```python
from build123d import *

# Parameters (mm, degrees)
SKETCH_1_W                  = 82
SKETCH_1_H                  = 160
EXTRUDE_1_DEPTH             = 50
SKETCH_2_W                  = 79.5
SKETCH_2_H                  = 47.5
CUT_EXTRUDE_1_DEPTH         = 187.611896727
CUT_EXTRUDE_6_DEPTH         = 186.95765647
CUT_EXTRUDE_9_DEPTH         = 187.611896727
CUT_EXTRUDE_10_DEPTH        = 187.611896727
CUT_EXTRUDE_11_DEPTH        = 187.611896727
CUT_EXTRUDE_12_DEPTH        = 187.611896727
CUT_EXTRUDE_13_DEPTH        = 187.611896727
CUT_EXTRUDE_14_DEPTH        = 187.611896727
CUT_EXTRUDE_15_DEPTH        = 187.611896727
CUT_EXTRUDE_16_DEPTH        = 187.611896727
CUT_EXTRUDE_17_DEPTH        = 187.611896727
CUT_EXTRUDE_18_DEPTH        = 187.611896727
CUT_EXTRUDE_19_DEPTH        = 187.611896727
CUT_EXTRUDE_20_DEPTH        = 187.611896727
HOLE_WIZARD_3_4_3_4_1_D     = 3.4
HOLE_WIZARD_3_4_3_4_1_DEPTH = 50
HOLE_WIZARD_3_2_3_2_2_D     = 3.2
HOLE_WIZARD_3_2_3_2_2_DEPTH = 82
HOLE_WIZARD_5_0_5_1_D       = 5
HOLE_WIZARD_5_0_5_1_DEPTH   = 50
FILLET_1_R                  = 0.5
FILLET_2_R                  = 2
FILLET_3_R                  = 5
SKETCH_30_R                 = 1.6
CUT_EXTRUDE_21_DEPTH        = 10
SKETCH_31_R                 = 1.6
CUT_EXTRUDE_22_DEPTH        = 186.52695222


with BuildPart() as part:
    # 草图1 → 凸台-拉伸1 (new body)
    with BuildSketch(Plane(origin=(0, 0, -50), x_dir=(-1, 0, 0), z_dir=(0, 0, -1))):
        with Locations((-41, 80)):
            Rectangle(SKETCH_1_W, SKETCH_1_H)
    extrude(amount=-EXTRUDE_1_DEPTH)

    # 草图2 → 切除-拉伸1 (cut, through all)
    with BuildSketch(Plane(origin=(0, 160, 0), x_dir=(-1, 0, 0), z_dir=(0, 1, 0))):
        with Locations((-39.75, -26.25)):
            Rectangle(SKETCH_2_W, SKETCH_2_H)
    extrude(amount=-CUT_EXTRUDE_1_DEPTH, mode=Mode.SUBTRACT)

    # 草图7 → 切除-拉伸6 (cut, through all)
    with BuildSketch(Plane(origin=(0, 0, -2.5), x_dir=(-1, 0, 0), z_dir=(0, 0, -1))):
        with BuildLine():
            Line((-68, 20), (-38, 20))
            ThreePointArc((-38, 20), (-36.4, 21.6), (-38, 23.2))
            Line((-38, 23.2), (-68, 23.2))
            ThreePointArc((-68, 23.2), (-69.6, 21.6), (-68, 20))
        make_face()
    extrude(amount=-CUT_EXTRUDE_6_DEPTH, mode=Mode.SUBTRACT)

    # 草图10 → 切除-拉伸9 (cut, through all)
    with BuildSketch(Plane(origin=(82, 0, 0), x_dir=(0, 0, -1), z_dir=(1, 0, 0))):
        with BuildLine():
            Line((20.690598923, 80), (16.690598923, 86.92820323))
            ThreePointArc((16.690598923, 86.92820323), (13.629378785, 80), (16.690598923, 73.07179677))
            Line((16.690598923, 73.07179677), (20.690598923, 80))
        make_face()
    extrude(amount=-CUT_EXTRUDE_9_DEPTH, mode=Mode.SUBTRACT)

    # 草图11 → 切除-拉伸10 (cut, through all)
    with BuildSketch(Plane(origin=(82, 0, 0), x_dir=(0, 0, -1), z_dir=(1, 0, 0))):
        with BuildLine():
            Line((20.154700538, 88.92820323), (24.154700538, 82))
            Line((24.154700538, 82), (32.154700538, 82))
            ThreePointArc((32.154700538, 82), (27.685310607, 88.115196021), (20.154700538, 88.92820323))
        make_face()
    extrude(amount=-CUT_EXTRUDE_10_DEPTH, mode=Mode.SUBTRACT)

    # 草图12 → 切除-拉伸11 (cut, through all)
    with BuildSketch(Plane(origin=(82, 0, 0), x_dir=(0, 0, -1), z_dir=(1, 0, 0))):
        with BuildLine():
            Line((24.154700538, 78), (20.154700538, 71.07179677))
            ThreePointArc((20.154700538, 71.07179677), (27.685310607, 71.884803979), (32.154700538, 78))
            Line((32.154700538, 78), (24.154700538, 78))
        make_face()
    extrude(amount=-CUT_EXTRUDE_11_DEPTH, mode=Mode.SUBTRACT)

    # 草图13 → 切除-拉伸12 (cut, through all)
    with BuildSketch(Plane(origin=(82, 0, 0), x_dir=(0, 0, -1), z_dir=(1, 0, 0))):
        with BuildLine():
            Line((36, 21.2), (14, 21.2))
            ThreePointArc((14, 21.2), (12.4, 19.6), (14, 18))
            Line((14, 18), (36, 18))
            ThreePointArc((36, 18), (37.6, 19.6), (36, 21.2))
        make_face()
    extrude(amount=-CUT_EXTRUDE_12_DEPTH, mode=Mode.SUBTRACT)

    # 草图14 → 切除-拉伸13 (cut, through all)
    with BuildSketch(Plane(origin=(82, 0, 0), x_dir=(0, 0, -1), z_dir=(1, 0, 0))):
        with BuildLine():
            Line((36, 31.2), (14, 31.2))
            ThreePointArc((14, 31.2), (12.4, 29.6), (14, 28))
            Line((14, 28), (36, 28))
            ThreePointArc((36, 28), (37.6, 29.6), (36, 31.2))
        make_face()
    extrude(amount=-CUT_EXTRUDE_13_DEPTH, mode=Mode.SUBTRACT)

    # 草图15 → 切除-拉伸14 (cut, through all)
    with BuildSketch(Plane(origin=(82, 0, 0), x_dir=(0, 0, -1), z_dir=(1, 0, 0))):
        with BuildLine():
            Line((36, 41.2), (14, 41.2))
            ThreePointArc((14, 41.2), (12.4, 39.6), (14, 38))
            Line((14, 38), (36, 38))
            ThreePointArc((36, 38), (37.6, 39.6), (36, 41.2))
        make_face()
    extrude(amount=-CUT_EXTRUDE_14_DEPTH, mode=Mode.SUBTRACT)

    # 草图16 → 切除-拉伸15 (cut, through all)
    with BuildSketch(Plane(origin=(82, 0, 0), x_dir=(0, 0, -1), z_dir=(1, 0, 0))):
        with BuildLine():
            Line((36, 51.2), (14, 51.2))
            ThreePointArc((14, 51.2), (12.4, 49.6), (14, 48))
            Line((14, 48), (36, 48))
            ThreePointArc((36, 48), (37.6, 49.6), (36, 51.2))
        make_face()
    extrude(amount=-CUT_EXTRUDE_15_DEPTH, mode=Mode.SUBTRACT)

    # 草图17 → 切除-拉伸16 (cut, through all)
    with BuildSketch(Plane(origin=(82, 0, 0), x_dir=(0, 0, -1), z_dir=(1, 0, 0))):
        with BuildLine():
            Line((36, 112), (14, 112))
            ThreePointArc((14, 112), (12.4, 110.4), (14, 108.8))
            Line((14, 108.8), (36, 108.8))
            ThreePointArc((36, 108.8), (37.6, 110.4), (36, 112))
        make_face()
    extrude(amount=-CUT_EXTRUDE_16_DEPTH, mode=Mode.SUBTRACT)

    # 草图18 → 切除-拉伸17 (cut, through all)
    with BuildSketch(Plane(origin=(82, 0, 0), x_dir=(0, 0, -1), z_dir=(1, 0, 0))):
        with BuildLine():
            Line((36, 122), (14, 122))
            ThreePointArc((14, 122), (12.4, 120.4), (14, 118.8))
            Line((14, 118.8), (36, 118.8))
            ThreePointArc((36, 118.8), (37.6, 120.4), (36, 122))
        make_face()
    extrude(amount=-CUT_EXTRUDE_17_DEPTH, mode=Mode.SUBTRACT)

    # 草图19 → 切除-拉伸18 (cut, through all)
    with BuildSketch(Plane(origin=(82, 0, 0), x_dir=(0, 0, -1), z_dir=(1, 0, 0))):
        with BuildLine():
            Line((36, 132), (14, 132))
            ThreePointArc((14, 132), (12.4, 130.4), (14, 128.8))
            Line((14, 128.8), (36, 128.8))
            ThreePointArc((36, 128.8), (37.6, 130.4), (36, 132))
        make_face()
    extrude(amount=-CUT_EXTRUDE_18_DEPTH, mode=Mode.SUBTRACT)

    # 草图20 → 切除-拉伸19 (cut, through all)
    with BuildSketch(Plane(origin=(82, 0, 0), x_dir=(0, 0, -1), z_dir=(1, 0, 0))):
        with BuildLine():
            Line((36, 142), (14, 142))
            ThreePointArc((14, 142), (12.4, 140.4), (14, 138.8))
            Line((14, 138.8), (36, 138.8))
            ThreePointArc((36, 138.8), (37.6, 140.4), (36, 142))
        make_face()
    extrude(amount=-CUT_EXTRUDE_19_DEPTH, mode=Mode.SUBTRACT)

    # 草图21 → 切除-拉伸20 (cut, through all)
    with BuildSketch(Plane.XY):
        with BuildLine():
            Line((68, 140), (38, 140))
            ThreePointArc((38, 140), (36.4, 138.4), (38, 136.8))
            Line((38, 136.8), (68, 136.8))
            ThreePointArc((68, 136.8), (69.6, 138.4), (68, 140))
        make_face()
    extrude(amount=-CUT_EXTRUDE_20_DEPTH, mode=Mode.SUBTRACT)

    # Ø3.4 (3.4) 直径孔1
    with Locations(Plane.XY):
        with Locations((31.5, 154), (42, 154), (71.5, 154), (71.5, 6), (42, 6), (31.5, 6), (19, 8), (19, 15), (19, 145), (19, 152)):
            Hole(HOLE_WIZARD_3_4_3_4_1_D / 2, depth=HOLE_WIZARD_3_4_3_4_1_DEPTH)

    # Ø3.2 (3.2) 直径孔2
    with Locations(Plane(origin=(82, 0, 0), x_dir=(0, 0, -1), z_dir=(1, 0, 0))):
        with Locations((9.5, 150), (17.5, 150), (25.5, 150), (33.5, 150), (41.5, 150), (41.5, 10), (33.5, 10), (25.5, 10), (17.5, 10), (10.5, 90), (23, 100), (35.5, 90), (9.5, 10), (35.5, 70), (23, 60), (10.5, 70)):
            Hole(HOLE_WIZARD_3_2_3_2_2_D / 2, depth=HOLE_WIZARD_3_2_3_2_2_DEPTH)

    # Ø5.0 (5) 直径孔1
    with Locations(Plane.XY):
        with Locations((6, 17), (6, 42), (6, 118), (6, 143)):
            Hole(HOLE_WIZARD_5_0_5_1_D / 2, depth=HOLE_WIZARD_5_0_5_1_DEPTH)

    # 圆角1
    fillet_1_edges = [part.edges().sort_by_distance(p)[0] for p in [
        (79.5, 80, -2.5),
    ]]
    fillet(fillet_1_edges, radius=FILLET_1_R)

    # 圆角2
    fillet_2_edges = [part.edges().sort_by_distance(p)[0] for p in [
        (82, 80, 0),
    ]]
    fillet(fillet_2_edges, radius=FILLET_2_R)

    # 圆角3
    fillet_3_edges = [part.edges().sort_by_distance(p)[0] for p in [
        (80.75, 160, -50),
        (80.75, 0, -50),
        (0, 160, -1.25),
        (0, 0, -1.25),
    ]]
    fillet(fillet_3_edges, radius=FILLET_3_R)

    # 草图30 → 切除-拉伸21 (cut)
    with BuildSketch(Plane(origin=(0, 0, -2.5), x_dir=(-1, 0, 0), z_dir=(0, 0, -1))):
        with Locations((-40, 59)):
            Circle(SKETCH_30_R)
        with Locations((-40, 53)):
            Circle(SKETCH_30_R)
        with Locations((-30, 59)):
            Circle(SKETCH_30_R)
        with Locations((-30, 53)):
            Circle(SKETCH_30_R)
        with Locations((-40, 107)):
            Circle(SKETCH_30_R)
        with Locations((-30, 107)):
            Circle(SKETCH_30_R)
        with Locations((-30, 101)):
            Circle(SKETCH_30_R)
        with Locations((-40, 101)):
            Circle(SKETCH_30_R)
    extrude(amount=-CUT_EXTRUDE_21_DEPTH, mode=Mode.SUBTRACT)

    # 草图31 → 切除-拉伸22 (cut, through all)
    with BuildSketch(Plane.ZY.offset(-79.5)):
        with Locations((-40, 32.35)):
            Circle(SKETCH_31_R)
        with Locations((-40, 22.35)):
            Circle(SKETCH_31_R)
        with Locations(Location((-40, 137.65, 0), (0, 0, 180))):
            Circle(SKETCH_31_R)
        with Locations(Location((-40, 127.65, 0), (0, 0, 180))):
            Circle(SKETCH_31_R)
    extrude(amount=-CUT_EXTRUDE_22_DEPTH, mode=Mode.SUBTRACT)


solid = part.part
```
Check sheet for the modelled part. Datum: model origin and axes. Units: mm. A direction names the side the tool comes from. Give positions to 0.01 mm unless a question says otherwise; leave off trailing zeros. Write each loop counter-clockwise with the first axis right and the second up, starting at its lowest first coordinate (ties: lowest second). Pieces come first, ordered by that corner, then holes. Notation, with made-up numbers: (22.25, 4) - (36.25, 4) arc R11 cw to (36.25, 8) - close; hole circle Ø6 at (35, 78). An arc over 180 degrees is marked (long way). Answer as a JSON object with one key per item and string values. Group by question number.
1) Sectioned sample at C-C (x = 25). Record the cut outline in (y, z), then the cut area to 3 significant figures.
2) Depth check by flat-ended pin: P1, Ø12, axis at y = 64.5, z = -28, coming from the -X side; P2, Ø1.5, axis at x = 15, y = 83.5, coming from the -Z side; P3, Ø2, axis at x = 42, y = 154, coming from the +Z side. Enter the tip coordinate at first touch or a pass-through.
3) Sectioned sample at A-A (x = 62). Record the cut outline in (y, z), then the cut area to 3 significant figures.
4) Access from +Z, -Z, +X, -X, +Y, -Y to the whole of each face (thin tool, end or side, straight path). Record for faces 1 (the face through (6.33, 145.48, -1.27)), 2 (the face through (80.768, 83.416, -18.719)), 3 (the face through (40, 81, -2.5)).
5) Thickness scan on probe 1 along Z at (x, y) = (80, 90); probe 2 along Z at (x, y) = (80, 150); probe 3 along X at (y, z) = (154, -1). Record the ranges inside material, lowest first. Write a range as from..to.
6) Release check for a two-part mould opening along X. For faces 4 (the face through (80.732, 126.064, -39.792)), 5 (the face through (2, 1, -1)), 6 (the face through (6.54, 39.56, -1.27)) record: pulls with the +X half, pulls with the -X half, needs draft (parallel to the pull), parting line crosses it, or undercut.
7) Sectioned sample at B-B (z = -30). Give the number of separate pieces and of enclosed holes in the cut face, then the cut area to 3 significant figures.
Geometry results:
{
 "1": {"outline": "(0, -2.5) - (160, -2.5) - (160, 0) - (0, 0) - close", "area": "400 mm^2"},
 "2": {"P1": "stops at x = 79.5", "P2": "stops at z = -2.5", "P3": "passes through"},
 "3": {"outline": "(0, -2.5) - (20, -2.5) - (20, 0) - (0, 0) - close; (23.2, -2.5) - (136.8, -2.5) - (136.8, 0) - (23.2, 0) - close; (140, -2.5) - (160, -2.5) - (160, 0) - (140, 0) - close", "area": "384 mm^2"},
 "4": {"face 1": "+Z, -Z", "face 2": "+X, -X", "face 3": "-Z, -X, +Y, -Y"},
 "5": {"probe 1": "z = -50..-37.1, -33.9..-12.1, -8.9..0", "probe 2": "z = -50..-43.1, -39.9..-35.1, -31.9..-27.1, -23.9..-19.1, -15.9..-11.1, -7.9..0", "probe 3": "x = 0..29.8, 33.2..40.3, 43.7..69.8, 73.2..81.73"},
 "6": {"face 4": "needs draft", "face 5": "pulls with the -X half", "face 6": "undercut"},
 "7": {"separate pieces": "11", "enclosed holes": "0", "area": "315 mm^2"}
}
